```python
from build123d import *

# Parameters (mm, degrees)
SKETCH1_W           = 66
SKETCH1_H           = 67
BOSS_EXTRUDE1_DEPTH = 2
SKETCH2_W           = 66
SKETCH2_H           = 6
BOSS_EXTRUDE2_DEPTH = 9
SKETCH4_R           = 1.45
CUT_EXTRUDE1_DEPTH  = 3
SKETCH5_R           = 1.05
CUT_EXTRUDE2_DEPTH  = 3
CHAMFER1_SIZE       = 0.75


with BuildPart() as part:
    # Sketch1 → Boss-Extrude1 (new body)
    with BuildSketch(Plane(origin=(0, 0, 0), x_dir=(1, 0, 0), z_dir=(0, 1, 0))):
        with Locations((33, 33.5)):
            Rectangle(SKETCH1_W, SKETCH1_H)
    extrude(amount=BOSS_EXTRUDE1_DEPTH)

    # Sketch2 → Boss-Extrude2 (add)
    with BuildSketch(Plane(origin=(0, 2, 0), x_dir=(1, 0, 0), z_dir=(0, 1, 0))):
        with Locations((33, 64)):
            Rectangle(SKETCH2_W, SKETCH2_H)
        Polygon((17.257397729, 6), (66, 6), (66, 0), (0, 0), (0, 6), (12.5, 6), (12.5, 4.5), (17.257397729, 4.5), align=None)
    extrude(amount=BOSS_EXTRUDE2_DEPTH)

    # Sketch4 → Cut-Extrude1 (cut)
    with BuildSketch(Plane(origin=(0, 11, 0), x_dir=(1, 0, 0), z_dir=(0, 1, 0))):
        with Locations(Location((3, 64, 0), (0, 0, 270))):
            Circle(SKETCH4_R)
        with Locations(Location((63, 64, 0), (0, 0, 270))):
            Circle(SKETCH4_R)
        with Locations(Location((63, 3, 0), (0, 0, 270))):
            Circle(SKETCH4_R)
        with Locations(Location((3, 3, 0), (0, 0, 270))):
            Circle(SKETCH4_R)
    extrude(amount=-CUT_EXTRUDE1_DEPTH, mode=Mode.SUBTRACT)

    # Sketch5 → Cut-Extrude2 (cut)
    with BuildSketch(Plane(origin=(0, 8, 0), x_dir=(1, 0, 0), z_dir=(0, 1, 0))):
        with Locations(Location((3, 64, 0), (0, 0, 270))):
            Circle(SKETCH5_R)
        with Locations(Location((63, 64, 0), (0, 0, 270))):
            Circle(SKETCH5_R)
        with Locations(Location((63, 3, 0), (0, 0, 270))):
            Circle(SKETCH5_R)
        with Locations(Location((3, 3, 0), (0, 0, 270))):
            Circle(SKETCH5_R)
    extrude(amount=-CUT_EXTRUDE2_DEPTH, mode=Mode.SUBTRACT)

    # Chamfer1
    chamfer1_edges = [part.edges().sort_by_distance(p)[0] for p in [
        (33, 2, -61),
        (33, 11, -61),
        (33, 11, -67),
        (41.628698864, 2, -6),
        (6.25, 2, -6),
        (33, 11, 0),
        (41.628698864, 11, -6),
        (6.25, 11, -6),
        (33, 0, -67),
        (33, 0, 0),
    ]]
    chamfer(chamfer1_edges, length=CHAMFER1_SIZE)


solid = part.part
```
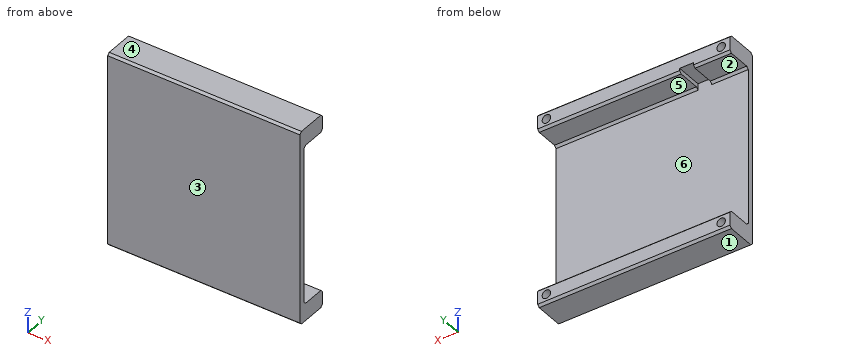
Here's how the part is built. I have some questions about the finished solid (model axes, mm). Face numbers are marked on the shaded views. A direction names the side the tool comes from. Coordinates: 2 decimals unless noted, no trailing zeros. Order: outer loops, then holes, each group sorted by start corner. A loop starts at its lowest first (then second) coordinate and runs counter-clockwise, first axis right, second up. Notation, with made-up numbers: M 44.5,26.25 L 93.5,26.25 A19 cw 93.5,47.25 Z; hole C 9.25,-6 d7. An arc over 180 degrees is marked long. Answer as a JSON object with one key per item and string values. Group by question number.
(1) Suppose I cut it at A-A, the plane y = 7. Please give me the cut outline in (x, z), then the cut area to 3 significant figures.
(2) Suppose I cut it at B-B, the plane x = 59.5. Please give me the cut outline in (y, z).
(3) Which directions (+Z, -Z, +X, -X, +Y, -Y) give clear straight access to the entire face, cutting with the end or side of a thin tool? Please do the marked faces 1 and 2.
(4) For pin 1 (1.9 mm diameter, centred on x = 63, z = -64, fed in from +Y); pin 2 (8 mm diameter, centred on x = 15.5, z = -19.5, fed in from +Y); pin 3 (2.5 mm diameter, centred on x = 3, z = -3, fed in from +Y), each with a flat end and sliding along its axis, tell me the tip position at first contact or that it passes through.
(5) If we mould it in two halves opening along Z, with no side actions, what happens to the marked faces 3, 4, 5 and 6? For each: released by +Z, released by -Z, zero draft, split by the parting line, or undercut.
(6) I need wall thicknesses on probe 1 along X at (y, z) = (6.3, -64); probe 2 along X at (y, z) = (9.4, -64); probe 3 along Z at (x, y) = (56.5, 4.5). Which ranges of each line are inside material? Lowest first, please.
(7) Suppose I cut it at C-C, the plane z = -64. Please give me the cut outline in (x, y).
Values found:
{
 "1": {"outline": "M 0,-67 L 66,-67 L 66,-61 L 0,-61 Z; M 0,-6 L 12.5,-6 L 12.5,-4.5 L 17.26,-4.5 L 17.26,-6 L 66,-6 L 66,0 L 0,0 Z; hole C 3,-64 d2.1; hole C 3,-3 d2.1; hole C 63,-64 d2.1; hole C 63,-3 d2.1", "area": "771 mm^2"},
 "2": {"outline": "M 0,-66.25 L 0.75,-67 L 10.25,-67 L 11,-66.25 L 11,-61.75 L 10.25,-61 L 2.75,-61 L 2,-60.25 L 2,-6.75 L 2.75,-6 L 10.25,-6 L 11,-5.25 L 11,-0.75 L 10.25,0 L 0.75,0 L 0,-0.75 Z"},
 "3": {"face 1": "-Z, +X, -X, +Y, -Y", "face 2": "+X, -X, +Y"},
 "4": {"pin 1": "stops at y = 5", "pin 2": "stops at y = 2", "pin 3": "stops at y = 8"},
 "5": {"face 3": "zero draft", "face 4": "released by +Z", "face 5": "undercut", "face 6": "undercut"},
 "6": {"probe 1": "x = 0 to 1.95, 4.05 to 61.95, 64.05 to 66", "probe 2": "x = 0 to 1.55, 4.45 to 61.55, 64.45 to 66", "probe 3": "z = -67 to -61, -6 to 0"},
 "7": {"outline": "M 0,0 L 66,0 L 66,11 L 64.45,11 L 64.45,8 L 64.05,8 L 64.05,5 L 61.95,5 L 61.95,8 L 61.55,8 L 61.55,11 L 4.45,11 L 4.45,8 L 4.05,8 L 4.05,5 L 1.95,5 L 1.95,8 L 1.55,8 L 1.55,11 L 0,11 Z"}
}
